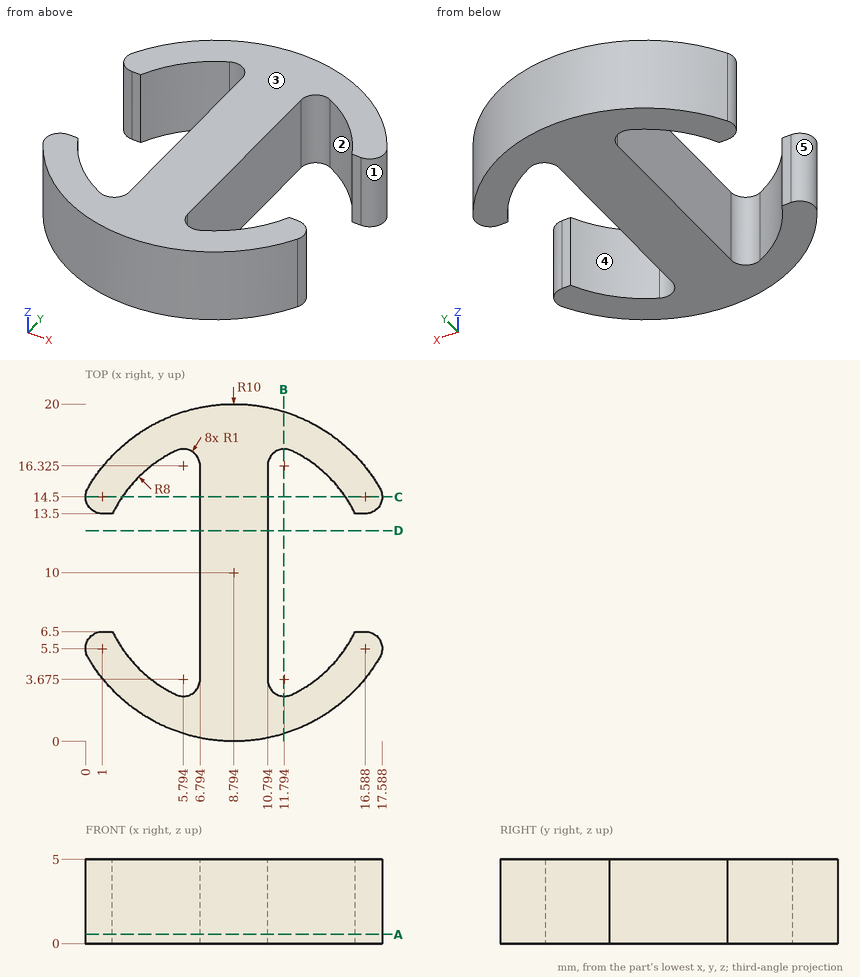
Print and shaded views of the part. All mm, measured from the part's lowest x, y and z. A direction names the side the tool comes from. Give positions to 0.01 mm unless a question says otherwise; leave off trailing zeros. Order: outer loops, then holes, each group sorted by start corner. A loop starts at its lowest first (then second) coordinate and runs counter-clockwise, first axis right, second up. Notation, with made-up numbers: (54, 51) - (67, 51) arc R31 ccw to (67, 80) - close; hole circle Ø6 at (-21.75, 42). An arc over 180 degrees is marked (long way). Use a Markdown table: item, result.
1) Two-plate mould, pull along X, no slides. Class the marked faces 3, 4 and 5: +X half, -X half, draft (parallel to the pull), parting line (faces both ways), or undercut.
Checked values:
| item | result |
|---|---|
| face 3 | draft |
| face 4 | undercut |
| face 5 | -X half |
2) Saw through at B-B on x = 11.75. List the corners of the cut face in (y, z).
Checked values:
| item | result |
|---|---|
| outline | (0.45, 0) - (2.68, 0) - (2.68, 5) - (0.45, 5) - close; (17.32, 0) - (19.55, 0) - (19.55, 5) - (17.32, 5) - close |
3) Flat gauge pins, fed straight in: P1, Ø0.5, axis at x = 1.5, z = 1.5, coming from the +Y side; P2, Ø0.5, axis at x = 16, z = 2.5, coming from the +Y side (1 decimal); P3, Ø2, axis at x = 13.5, y = 4, coming from the +Z side; P4, Ø2, axis at x = 15.5, z = 3, coming from the +Y side. Where does each tip first touch, or does it go through?
Checked values:
| item | result |
|---|---|
| P1 | y = 17.1 |
| P2 | y = 17.2 |
| P3 | z = 5 |
| P4 | y = 18.21 |
4) Probe L1, parallel to X at y = 3.25, z = 0.95 (1 decimal); L2, parallel to X at y = 5.25, z = 2.45 (1 decimal); L3, parallel to Y at x = 12.25, z = 1.25 (1 decimal). List the from-to ranges inside material, lowest first. Write a range as from..to.
Checked values:
| item | result |
|---|---|
| L1 | 1.4..4.5, 6.7..10.9, 13.1..16.2 |
| L2 | 0..2.4, 6.8..10.8, 15.2..17.6 |
| L3 | 0.6..2.8, 17.2..19.4 |
5) Saw through at D-D on y = 12.5. List the corners of the cut face in (x, z) (1 decimal), plus the area to 3 significant figures.
Checked values:
| item | result |
|---|---|
| outline | (6.8, 0) - (10.8, 0) - (10.8, 5) - (6.8, 5) - close |
| area | 20.0 mm² |
6) 3-axis set-ups, long thin cutter, end or side, ignore diameter. For the marked faces 1 and 2: which of +Z, -Z, +X, -X, +Y, -Y reach the whole face in a straight line?
Checked values:
| item | result |
|---|---|
| face 1 | +Z, -Z, +X |
| face 2 | +Z, -Z |
7) Saw through at A-A on z = 0.55. List the corners of the cut face in (x, y) (1 decimal).
Checked values:
| item | result |
|---|---|
| outline | (0.1, 5) arc R10 ccw to (17.5, 5) arc R1 ccw to (16.6, 6.5) - (16, 6.5) arc R8 cw to (12.2, 2.8) arc R1 cw to (10.8, 3.7) - (10.8, 16.3) arc R1 cw to (12.2, 17.2) arc R8 cw to (16, 13.5) - (16.6, 13.5) arc R1 ccw to (17.5, 15) arc R10 ccw to (0.1, 15) arc R1 ccw to (1, 13.5) - (1.6, 13.5) arc R8 cw to (5.4, 17.2) arc R1 cw to (6.8, 16.3) - (6.8, 3.7) arc R1 cw to (5.4, 2.8) arc R8 cw to (1.6, 6.5) - (1, 6.5) arc R1 ccw to start |
8) Saw through at C-C on y = 14.5. List the corners of the cut face in (x, z) (1 decimal), plus the area to 3 significant figures.
Checked values:
| item | result |
|---|---|
| outline | (0, 0) - (2.2, 0) - (2.2, 5) - (0, 5) - close; (6.8, 0) - (10.8, 0) - (10.8, 5) - (6.8, 5) - close; (15.4, 0) - (17.6, 0) - (17.6, 5) - (15.4, 5) - close |
| area | 41.8 mm² |
